Read the model definition and answer for the solid it produces. Units are mm, in the model's axes. Face numbers are marked on the shaded views. A direction names the side the tool comes from. Round coordinates to 2 decimals unless told otherwise and drop trailing zeros. Order: outer loops, then holes, each group sorted by start corner. A loop starts at its lowest first (then second) coordinate and runs counter-clockwise, first axis right, second up. Notation, with made-up numbers: (-16, 48.5) - (36, 48.5) arc R9 cw to (36, 61.5) - close; hole circle Ø2 at (88.5, 73.5). An arc over 180 degrees is marked (long way). Answer as a JSON object with one key per item and string values. Group by question number.
Q1. A cutting plane is placed at B-B on x = -10. Determine the outline of the cut face in (y, z), and give its area (3 significant figures).
Q2. A cutting plane is placed at A-A on z = 14. Determine the outline of the cut face in (x, y), and give its area (3 significant figures).
Q3. A tool of negligible diameter and unlimited length cuts with its end or side. For the marked faces 1 and 2, from which of +Z, -Z, +X, -X, +Y, -Y can it reach the whole face along a straight path? Write none if from no direction.
Q4. Consider line 1 (Y direction, x = -10, z = 29.05); line 2 (Z direction, x = -12.75, y = 6.5); line 3 (X direction, y = 16, z = 16.25). Determine where each line is inside the solid, lowest interval first.
Q5. Given pin 1 Ø1 at (x, y) = (-5, 12) entering from -Z; pin 2 Ø1 at (y, z) = (7, 25.5) entering from -X, each flat-ended and moving along its own axis, determine where each tip first touches the part or whether it passes through.
Q6. A cutting plane is placed at D-D on y = 4.75. Determine the outline of the cut face in (x, z), and give its area (3 significant figures).
Q7. A cutting plane is placed at C-C on y = 9.5. Determine the outline of the cut face in (x, z).
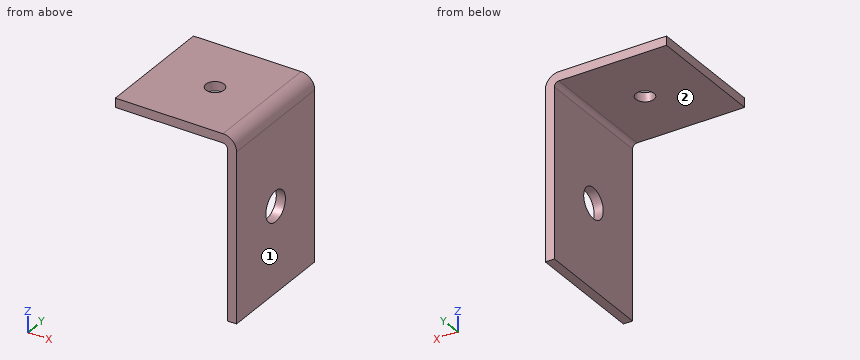
```python
from build123d import *

# Parameters (mm, degrees)
BASE_FLANGE1_DEPTH              = 20
F_5_0MM_PRESS_DOWEL_HOLE1_D     = 5
F_3_0MM_PRESS_DOWEL_HOLE1_D     = 3
F_3_0MM_PRESS_DOWEL_HOLE2_D     = 3
F_3_0MM_PRESS_DOWEL_HOLE2_DEPTH = 6
F_3_0MM_PRESS_DOWEL_HOLE2_TIP   = 0.901290929


# Sheet-metal steps are written as plain solids
with BuildPart() as part:
    # Sketch1 → Base-Flange1 (new body)
    with BuildSketch(Plane(origin=(0, 0, 0), x_dir=(1, 0, 0), z_dir=(0, 1, 0))):
        with BuildLine():
            Line((0, 0), (0, -27.7634))
            ThreePointArc((0, -27.7634), (-0.655084973, -29.344915027), (-2.2366, -30))
            Line((-2.2366, -30), (-20, -30))
            Line((-20, -30), (-20, -28.5))
            Line((-20, -28.5), (-2.2366, -28.5))
            ThreePointArc((-2.2366, -28.5), (-1.715745145, -28.284254855), (-1.5, -27.7634))
            Line((-1.5, -27.7634), (-1.5, 0))
            Line((-1.5, 0), (0, 0))
        make_face()
    extrude(amount=BASE_FLANGE1_DEPTH)

    # Ø5.0mm Press Dowel Hole1 (through all)
    with Locations(Plane(origin=(0, 0, 0), x_dir=(0, 0, -1), z_dir=(1, 0, 0))):
        with Locations((-14, 10)):
            Hole(F_5_0MM_PRESS_DOWEL_HOLE1_D / 2)

    # Ø3.0mm Press Dowel Hole1 (through all)
    with Locations(Plane(origin=(0, 0, 28.5), x_dir=(-1, 0, 0), z_dir=(0, 0, -1))):
        with Locations((10, 10)):
            Hole(F_3_0MM_PRESS_DOWEL_HOLE1_D / 2)

    # Ø3.0mm Press Dowel Hole2
    with Locations(Plane(origin=(-166.531359221, -210.525513363, 30), x_dir=(0, 1, 0), z_dir=(0, 0, -1))):
        with Locations((220.525513363, 156.531359221), (102.525513363, 181.531359221), (102.525513363, 271.531359221), (89.19270005, 226.531359221), (210.525513363, 317.793651488), (230.525513363, 317.793651488), (252.525513363, 320.462332131), (232.525513363, 300.462332131), (252.525513363, 132.600386311), (232.525513363, 152.600386311), (111.286271896, 136.531359221), (91.286271896, 136.531359221), (41.525513363, 196.432813402), (13.525513363, 196.432813402), (41.525513363, 138.767959221), (13.525513363, 138.767959221), (41.525513363, 256.62990504), (13.525513363, 256.62990504), (41.525513363, 314.294759221), (13.525513363, 314.294759221)):
            Hole(F_3_0MM_PRESS_DOWEL_HOLE2_D / 2, depth=F_3_0MM_PRESS_DOWEL_HOLE2_DEPTH)
            with Locations((0, 0, -(F_3_0MM_PRESS_DOWEL_HOLE2_DEPTH + F_3_0MM_PRESS_DOWEL_HOLE2_TIP / 2))):  # 118° drill point
                Cone(0, F_3_0MM_PRESS_DOWEL_HOLE2_D / 2, F_3_0MM_PRESS_DOWEL_HOLE2_TIP, mode=Mode.SUBTRACT)


solid = part.part
```
Result set:
{
 "1": {"outline": "(0, 28.5) - (8.5, 28.5) - (8.5, 30) - (0, 30) - close; (11.5, 28.5) - (20, 28.5) - (20, 30) - (11.5, 30) - close", "area": "25.5 mm²"},
 "2": {"outline": "(-1.5, 0) - (0, 0) - (0, 7.5) - (-1.5, 7.5) - close; (-1.5, 12.5) - (0, 12.5) - (0, 20) - (-1.5, 20) - close", "area": "22.5 mm²"},
 "3": {"face 1": "+Z, -Z, +X, +Y, -Y", "face 2": "-Z, -X, +Y, -Y"},
 "4": {"line 1": "y = 0 to 8.5, 11.5 to 20", "line 2": "z = 28.5 to 30", "line 3": "x = -1.5 to 0"},
 "5": {"pin 1": "stops at z = 28.5", "pin 2": "stops at x = -1.5"},
 "6": {"outline": "(-20, 28.5) - (-2.24, 28.5) arc R0.74 cw to (-1.5, 27.76) - (-1.5, 0) - (0, 0) - (0, 27.76) arc R2.24 ccw to (-2.24, 30) - (-20, 30) - close", "area": "71.8 mm²"},
 "7": {"outline": "(-20, 28.5) - (-11.41, 28.5) - (-11.41, 30) - (-20, 30) - close; (-8.59, 28.5) - (-2.24, 28.5) arc R0.74 cw to (-1.5, 27.76) - (-1.5, 16.45) - (0, 16.45) - (0, 27.76) arc R2.24 ccw to (-2.24, 30) - (-8.59, 30) - close; (-1.5, 0) - (0, 0) - (0, 11.55) - (-1.5, 11.55) - close"}
}
